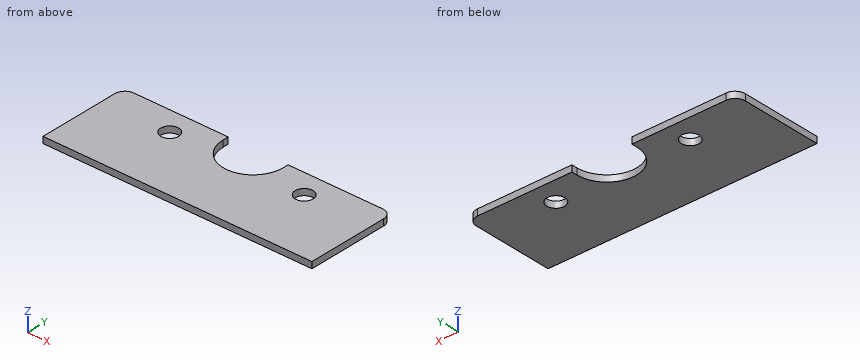
```python
from build123d import *

# Parameters (mm, degrees)
BOSS_EXTRUDE1_DEPTH  = 1.5875
M4_CLEARANCE_HOLE1_D = 4.5
FILLET1_R            = 2.54


with BuildPart() as part:
    # Sketch1 → Boss-Extrude1 (new body)
    with BuildSketch(Plane.XY):
        with BuildLine():
            Line((-21.1688151, 32.012776561), (4.9971849, 32.012776561))
            Line((4.9971849, 32.012776561), (4.9971849, 30.603076561))
            ThreePointArc((4.9971849, 30.603076561), (12.4971849, 23.103076561), (19.9971849, 30.603076561))
            Line((19.9971849, 30.603076561), (19.9971849, 32.012776561))
            Line((19.9971849, 32.012776561), (46.1631849, 32.012776561))
            Line((46.1631849, 32.012776561), (46.1631849, 9.152776561))
            Line((46.1631849, 9.152776561), (-21.1688151, 9.152776561))
            Line((-21.1688151, 9.152776561), (-21.1688151, 32.012776561))
        make_face()
    extrude(amount=BOSS_EXTRUDE1_DEPTH)

    # M4 Clearance Hole1 (through all)
    with Locations(Plane.XY.offset(1.5875)):
        with Locations((-4.3358151, 26.012776561), (29.3301849, 26.012776561)):
            Hole(M4_CLEARANCE_HOLE1_D / 2)

    # Fillet1
    fillet1_edges = [part.edges().sort_by_distance(p)[0] for p in [
        (46.1631849, 32.012776561, 0.79375),
        (-21.1688151, 32.012776561, 0.79375),
    ]]
    fillet(fillet1_edges, radius=FILLET1_R)


solid = part.part
```
Verification items for the finished model (mm, model axes). Give positions to 0.01 mm unless a question says otherwise; leave off trailing zeros. Order: outer loops, then holes, each group sorted by start corner. A loop starts at its lowest first (then second) coordinate and runs counter-clockwise, first axis right, second up. Notation, with made-up numbers: M -15,32.5 L -10,32.5 A23 cw -10,42.5 Z; hole C 70,80.25 d8. An arc over 180 degrees is marked long. Answer in a Markdown table with one row per item. Add a question column.
Item 1: Gauge pin test, flat end, axial feed: pin 1 (0.7 mm diameter, centred on y = 31, z = 1, fed in from +X). Record the tip position at first contact, or that the pin passes through.
Item 2: Section check C-C, the plane z = 1.05. Enter the section's corners in (x, y).
Item 3: Scan lines: probe 1 along X at (y, z) = (25, 0.85); probe 2 along X at (y, z) = (27.25, 0.25); probe 3 along X at (y, z) = (30, 0.8). Record each from-to range of solid material in increasing order. Write a range as from..to.
Item 4: Section check D-D, the plane x = 9.5. Enter the section's corners in (y, z), and give its area (3 significant figures).
Item 5: Section check A-A, the plane x = -3. Enter the section's corners in (y, z).
Item 6: Section check B-B, the plane y = 25.25. Enter the section's corners in (x, z), and give its area (3 significant figures).
Filled sheet:
| question | item | result |
|---|---|---|
| 1 | pin 1 | stops at x = 45.87 |
| 2 | outline | M -21.17,9.15 L 46.16,9.15 L 46.16,29.47 A2.54 ccw 43.62,32.01 L 20,32.01 L 20,30.6 A7.5 cw 5,30.6 L 5,32.01 L -18.63,32.01 A2.54 ccw -21.17,29.47 Z; hole C -4.34,26.01 d4.5; hole C 29.33,26.01 d4.5 |
| 3 | probe 1 | x = -21.17..-6.34, -2.33..7.51, 17.48..27.32, 31.34..46.16 |
| 3 | probe 2 | x = -21.17..-6.22, -2.46..5.79, 19.21..27.45, 31.21..46.16 |
| 3 | probe 3 | x = -21.11..5.02, 19.97..46.11 |
| 4 | outline | M 9.15,0 L 23.73,0 L 23.73,1.59 L 9.15,1.59 Z |
| 4 | area | 23.1 mm^2 |
| 5 | outline | M 9.15,0 L 24.2,0 L 24.2,1.59 L 9.15,1.59 Z; M 27.82,0 L 32.01,0 L 32.01,1.59 L 27.82,1.59 Z |
| 6 | outline | M -21.17,0 L -6.45,0 L -6.45,1.59 L -21.17,1.59 Z; M -2.22,0 L 7.24,0 L 7.24,1.59 L -2.22,1.59 Z; M 17.75,0 L 27.21,0 L 27.21,1.59 L 17.75,1.59 Z; M 31.45,0 L 46.16,0 L 46.16,1.59 L 31.45,1.59 Z |
| 6 | area | 76.8 mm^2 |
